from build123d import *

# Parameters (mm, degrees)
BOSS_EXTRUDE1_DEPTH = 100
SHELL9_T            = -3
CUT_EXTRUDE1_DEPTH  = 1
CUT_EXTRUDE2_START  = -1
CUT_EXTRUDE2_DEPTH  = 1
SKETCH4_W           = 10
SKETCH4_H           = 10
BOSS_EXTRUDE2_DEPTH = 5
CUT_EXTRUDE5_DEPTH  = 10
SKETCH6_W           = 10.495090221
SKETCH6_H           = 10
BOSS_EXTRUDE3_DEPTH = 10
SKETCH7_W           = 10.495090221
SKETCH7_H           = 10
SKETCH7_R           = 4
CUT_EXTRUDE6_DEPTH  = 10
SKETCH8_R           = 5
BOSS_EXTRUDE4_DEPTH = 2
CUT_EXTRUDE7_DEPTH  = 2
CIRPATTERN1_COUNT   = 12
SKETCH10_R          = 3.401579871
SKETCH10_R_2        = 2.401579871
BOSS_EXTRUDE5_DEPTH = 1
FILLET2_R           = 0.5
FILLET3_R           = 0.5
CUT_EXTRUDE8_START  = -3
CUT_EXTRUDE8_DEPTH  = 3


with BuildPart() as part:
    # Sketch1 → Boss-Extrude1 (new body)
    with BuildSketch(Plane.XY):
        with BuildLine():
            Line((-20, 25), (20, 25))
            ThreePointArc((20, 25), (23.535533906, 23.535533906), (25, 20))
            Line((25, 20), (25, -20))
            ThreePointArc((25, -20), (23.535533906, -23.535533906), (20, -25))
            Line((20, -25), (-20, -25))
            ThreePointArc((-20, -25), (-23.535533906, -23.535533906), (-25, -20))
            Line((-25, -20), (-25, 20))
            ThreePointArc((-25, 20), (-23.535533906, 23.535533906), (-20, 25))
        make_face()
    extrude(amount=BOSS_EXTRUDE1_DEPTH)

    # Shell9
    shell9_openings = [part.faces().sort_by_distance(p)[0] for p in [
        (0, 0, 0),
    ]]
    offset(amount=SHELL9_T, openings=shell9_openings, kind=Kind.INTERSECTION)

    # Sketch2 → Cut-Extrude1 (cut)
    with BuildSketch(Plane.XY.offset(100)):
        with BuildLine():
            Line((24, -20), (24, 20))
            ThreePointArc((24, 20), (22.828427125, 22.828427125), (20, 24))
            Line((20, 24), (-20, 24))
            ThreePointArc((-20, 24), (-22.828427125, 22.828427125), (-24, 20))
            Line((-24, 20), (-24, -20))
            ThreePointArc((-24, -20), (-22.828427125, -22.828427125), (-20, -24))
            Line((-20, -24), (20, -24))
            ThreePointArc((20, -24), (22.828427125, -22.828427125), (24, -20))
        make_face()
    extrude(amount=-CUT_EXTRUDE1_DEPTH, mode=Mode.SUBTRACT)

    # Sketch3 → Cut-Extrude2 (cut)
    with BuildSketch(Plane(origin=(0, 0, 0), x_dir=(-1, 0, 0), z_dir=(0, 0, -1)).offset(CUT_EXTRUDE2_START)):
        with BuildLine():
            Line((-20, -24), (20, -24))
            ThreePointArc((20, -24), (22.828427125, -22.828427125), (24, -20))
            Line((24, -20), (24, 20))
            ThreePointArc((24, 20), (22.828427125, 22.828427125), (20, 24))
            Line((20, 24), (-20, 24))
            ThreePointArc((-20, 24), (-22.828427125, 22.828427125), (-24, 20))
            Line((-24, 20), (-24, -20))
            ThreePointArc((-24, -20), (-22.828427125, -22.828427125), (-20, -24))
        make_face()
    extrude(amount=CUT_EXTRUDE2_DEPTH, mode=Mode.SUBTRACT)

    # Sketch4 → Boss-Extrude2 (add)
    with BuildSketch(Plane(origin=(0, 25, 0), x_dir=(1, 0, 0), z_dir=(0, 1, 0))):
        with Locations((15, -53.049640043)):
            Rectangle(SKETCH4_W, SKETCH4_H)
    extrude(amount=BOSS_EXTRUDE2_DEPTH)

    # Sketch5 → Cut-Extrude5 (cut)
    with BuildSketch(Plane.XY.offset(58.049640043)):
        Polygon((10, 28.185422855), (20, 25), (20, 30), (10, 30), align=None)
    extrude(amount=-CUT_EXTRUDE5_DEPTH, mode=Mode.SUBTRACT)

    # Sketch6 → Boss-Extrude3 (add)
    with BuildSketch(Plane(origin=(9.072374427, 28.480910825, 0), x_dir=(0.9528264920711829, -0.3035155284451262, 0), z_dir=(0.3035155284451262, 0.9528264920711829, 0))):
        with Locations((6.22109652, -53.049640043)):
            Rectangle(SKETCH6_W, SKETCH6_H)
    extrude(amount=BOSS_EXTRUDE3_DEPTH)

    # Sketch7 → Cut-Extrude6 (cut)
    with BuildSketch(Plane(origin=(12.107529711, 38.009175746, 0), x_dir=(0.9528264920711829, -0.30351552844512614, 0), z_dir=(0.30351552844512614, 0.952826492071183, 0))):
        with Locations((6.22109652, -53.049640043)):
            Rectangle(SKETCH7_W, SKETCH7_H)
        with Locations(Location((6.221096519, -53.049640043, 0), (0, 0, 180))):
            Circle(SKETCH7_R, mode=Mode.SUBTRACT)
    extrude(amount=-CUT_EXTRUDE6_DEPTH, mode=Mode.SUBTRACT)

    # Sketch8 → Boss-Extrude4 (add)
    with BuildSketch(Plane(origin=(12.107529711, 38.009175746, 0), x_dir=(0.9528264920711829, -0.30351552844512614, 0), z_dir=(0.30351552844512614, 0.952826492071183, 0))):
        with Locations(Location((6.221096519, -53.049640043, 0), (0, 0, 180))):
            Circle(SKETCH8_R)
    extrude(amount=-BOSS_EXTRUDE4_DEPTH)

    # Sketch9 → Cut-Extrude7 (cut)
    with BuildSketch(Plane(origin=(12.107529711, 38.009175746, 0), x_dir=(0.9528264920711829, -0.30351552844512614, 0), z_dir=(0.30351552844512614, 0.952826492071183, 0))):
        with BuildLine():
            ThreePointArc((1.251860541, -52.495840627), (1.222824963, -53.18109898), (1.287841277, -53.863883686))
            Line((1.287841277, -53.863883686), (1.974013697, -53.750629555))
            ThreePointArc((1.974013697, -53.750629555), (1.919851851, -53.218142557), (1.932190971, -52.683050363))
            Line((1.932190971, -52.683050363), (1.251860541, -52.495840627))
        make_face()
    cut_extrude7 = extrude(amount=-CUT_EXTRUDE7_DEPTH, mode=Mode.SUBTRACT)

    # CirPattern1: Cut-Extrude7 ×12 about axis
    cirpattern1_axis = Axis((5.927625573, -1.888199398, 53.049640043), (0.30351552844512614, 0.9528264920711829, 0))
    for i in range(1, CIRPATTERN1_COUNT):
        add(cut_extrude7.rotate(cirpattern1_axis, i * 360 / CIRPATTERN1_COUNT), mode=Mode.SUBTRACT)

    # Sketch10 → Boss-Extrude5 (add)
    with BuildSketch(Plane(origin=(12.107529711, 38.009175746, 0), x_dir=(0.9528264920711829, -0.30351552844512614, 0), z_dir=(0.30351552844512614, 0.952826492071183, 0))):
        with Locations(Location((6.055914609, -52.898554166, 0), (0, 0, 180))):
            Circle(SKETCH10_R)
        with Locations(Location((6.055914609, -52.898554166, 0), (0, 0, 180))):
            Circle(SKETCH10_R_2, mode=Mode.SUBTRACT)
    extrude(amount=BOSS_EXTRUDE5_DEPTH)

    # Fillet2
    fillet2_edges = [part.edges().sort_by_distance(p)[0] for p in [
        (21.422396529, 36.091505803, 52.898554166),
    ]]
    fillet(fillet2_edges, radius=FILLET2_R)

    # Fillet3
    fillet3_edges = [part.edges().sort_by_distance(p)[0] for p in [
        (20.469570037, 36.395021331, 52.898554166),
    ]]
    fillet(fillet3_edges, radius=FILLET3_R - 0.0001)  # a hair under: the kernel refuses the full size

    # Sketch12 → Cut-Extrude8 (cut)
    with BuildSketch(Plane(origin=(0, 0, 1), x_dir=(-1, 0, 0), z_dir=(0, 0, -1)).offset(CUT_EXTRUDE8_START)):
        with BuildLine():
            Line((-20, -24), (20, -24))
            ThreePointArc((20, -24), (22.828427125, -22.828427125), (24, -20))
            Line((24, -20), (24, 20))
            ThreePointArc((24, 20), (22.828427125, 22.828427125), (20, 24))
            Line((20, 24), (-20, 24))
            ThreePointArc((-20, 24), (-22.828427125, 22.828427125), (-24, 20))
            Line((-24, 20), (-24, -20))
            ThreePointArc((-24, -20), (-22.828427125, -22.828427125), (-20, -24))
        make_face()
    extrude(amount=CUT_EXTRUDE8_DEPTH, mode=Mode.SUBTRACT)


solid = part.part
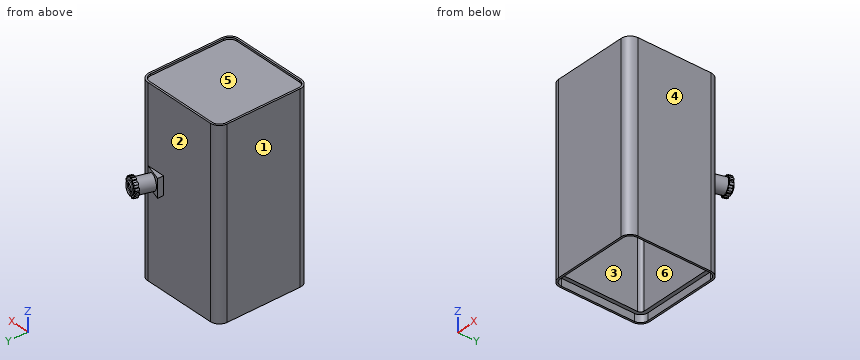
CAD build for the part. Positions are in the model's coordinates, mm. Face numbers are marked on the shaded views. A direction names the side the tool comes from. Round coordinates to 2 decimals unless told otherwise and drop trailing zeros. Write each loop counter-clockwise with the first axis right and the second up, starting at its lowest first coordinate (ties: lowest second). Pieces come first, ordered by that corner, then holes.
(1) 3-axis set-ups, long thin cutter, end or side, ignore diameter. For the marked faces 4, 5 and 6: which of +Z, -Z, +X, -X, +Y, -Y reach the whole face in a straight line?
(2) Slice it at B-B, the plane x = 6.5. Write the cut outline in (y, z).
(3) Drop flat-ended pins along their axis: P1, Ø12, axis at x = -9.5, z = 33.5, coming from the +Y side; P2, Ø24, axis at x = 7.5, y = -3, coming from the -Z side; P3, Ø12, axis at y = 25, z = 79, coming from the +X side; P4, Ø8, axis at x = -13.5, y = 5.5, coming from the +Z side. Give the stop position or say it passes through.
(4) Mould opens along X. For the marked faces 1, 2 and 3 say: pulls with the +X half, pulls with the -X half, needs draft (parallel to the pull), parting line crosses it, or undercut.
(5) Slice it at A-A, the plane z = 43.5. Write the cut outline in (x, y).
(6) Probe line 1 along Y through (x, z) = (0, 74); line 2 along Z through (x, y) = (3.5, -14.5). List the from-to ranges inside material, lowest first.
From the geometry:
1. face 4: +Z, -Z, +X, +Y, -Y
1. face 5: +Z
1. face 6: -Z
2. outline: (-25, 0) - (-24, 0) - (-24, 4) - (-22, 4) - (-22, 97) - (22, 97) - (22, 4) - (24, 4) - (24, 0) - (25, 0) - (25, 100) - (24, 100) - (24, 99) - (-24, 99) - (-24, 100) - (-25, 100) - close
3. P1: stops at y = 25
3. P2: stops at z = 97
3. P3: stops at x = 25
3. P4: stops at z = 99
4. face 1: pulls with the -X half
4. face 2: needs draft
4. face 3: undercut
5. outline: (-25, -20) arc R5 ccw to (-20, -25) - (20, -25) arc R5 ccw to (25, -20) - (25, 20) arc R5 ccw to (20, 25) - (-20, 25) arc R5 ccw to (-25, 20) - close; hole (-22, -20) arc R2 ccw to (-20, -22) - (20, -22) arc R2 ccw to (22, -20) - (22, 20) arc R2 ccw to (20, 22) - (-20, 22) arc R2 ccw to (-22, 20) - close
6. line 1: y = -25 to -22, 22 to 25
6. line 2: z = 97 to 99
